Autodesk Inventor part; units mm, degrees
ref_plane "Start Plane" through (0, 0, 5) normal (0, 0, 1) x (1, 0, 0)
ref_plane "End Plane" through (0, 0, 49.2474) normal (0, 0, 1) x (1, 0, 0)
ref_plane "Work Plane4" through (-5.9225, -101.2995, 61.7854) normal (0.3299, 0.1188, 0.9365) x (0.9438, -0.0202, -0.3299)
ref_plane "Start Plane" through (0, 0, 5) normal (0, 0, 1) x (1, 0, 0)
ref_plane "End Plane" through (0, 0, 49.2474) normal (0, 0, 1) x (1, 0, 0)
sketch "Sketch" plane through (0, 0, 0) normal (0, 0, 1) x (1, 0, 0)
  line L0 (5, -5) -> (-5, -5)
  line L1 (-5, -5) -> (-5, 5)
  line L2 (-5, 5) -> (5, 5)
  line L3 (5, 5) -> (5, -5)
  line L4 (-6, 0) -> (8, 0) construction
  line L5 (0, -30) -> (0, 40) construction
  line L6 (0, 54) -> (0, -44) construction
  line L7 (-9.2, 0) -> (13.2, 0) construction
  dimension "d0" = 10
  dimension "d1" = 10
  dimension "d4" = 5
  dimension "d5" = 5
extrude "Body" add sketch "Sketch" along normal up to surface (44.2474 mm away) from surface at 5
sketch "Sketch3" plane through (0, 0, 0) normal (0, 0, 1) x (1, 0, 0)
  line L0 (0, 0) -> (10, 0)
ref_plane "Work Plane3" through (0, 0, 0) normal (0, -1, 0) x (1, 0, 0)
sketch "Sketch4" plane through (0, 0, 0) normal (0, -1, 0) x (1, 0, 0)
  line L0 (-2, 5) -> (12, 5)
  line L1 (-2, 49.2474) -> (12, 49.2474)
  dimension "d9" = 44.2474
ref_plane "Work Plane4" through (-5.9225, -101.2995, 61.7854) normal (0.3299, 0.1188, 0.9365) x (0.9438, -0.0202, -0.3299)
split "Split1" plane through (-5.9225, -101.2995, 61.7854) removes the side toward (0.3299, 0.1188, 0.9365)
ref_plane "Work Plane5" through (-24.7397, 52.8201, 5) normal (0, 0, -1) x (-1, 0, 0)
split "Split2" plane through (-24.7397, 52.8201, 5) removes the side toward (0, 0, -1)
equation "\"d0\" = G_W"
equation "\"d1\" = G_H"
equation "\"d4\" = 0.5 * d1"
equation "\"d5\" = 0.5 * d0"
equation "\"d2\" = G_L"
equation "\"G_W\" = 10"
equation "\"G_H\" = 10"
equation "\"G_L\" = d9"
equation "\"G_OFFSET_START\" = -5"
equation "\"G_OFFSET_END\" = -8.2824"
equation "\"d6\" = -G_OFFSET_START"
equation "\"d7\" = G_OFFSET_END + B_L"
equation "\"B_L\" = 57.52978"
properties part number "ISO 1035/2 - 10 x 10 - 44.25" material "Steel, Mild"
Geometry: final body of the model. Coordinates: model frame, mm. Round coordinates to 2 decimals unless told otherwise and drop trailing zeros. Write each loop counter-clockwise with the first axis right and the second up, starting at its lowest first coordinate (ties: lowest second). Pieces come first, ordered by that corner, then holes. Notation, with made-up numbers: (74, -11.75) -> (98, -11.75) arc R31 cw to (98, 14.25) -> close; hole circle Ø3 at (59.25, 39.5). An arc over 180 degrees is marked (long way). Use CSV: the item, a comma, the result in double quotes. Start each with the question number.
Q1. Section B-B (x = 1.75). Return loops of the section in (y, z).
Q2. First-contact query: pin 1 Ø4 at (x, y) = (-0.5, 1.5) entering from +Z. Flat tip, straight axial feed; report the tip coordinate or a pass-through.
Q3. Section A-A (y = 1.5). Return loops of the section in (x, z).
Q4. Line query: L1, parallel to Z at x = -0.25, y = 3.5; L2, parallel to Z at x = 0.25, y = 3.5. Output: solid intervals per line, ascending.
Result sheet:
1,outline,"(-5, 5) -> (5, 5) -> (5, 45.6) -> (-5, 46.87) -> close"
2,pin 1,"z = 47.58"
3,outline,"(-5, 5) -> (5, 5) -> (5, 44.9) -> (-5, 48.42) -> close"
4,L1,"5 to 46.49"
4,L2,"5 to 46.32"
